For this review, take the finished solid that the model builds, in its own axes (mm). Face numbers are marked on the shaded views. Give positions to 0.01 mm unless a question says otherwise; leave off trailing zeros. Write each loop counter-clockwise with the first axis right and the second up, starting at its lowest first coordinate (ties: lowest second). Pieces come first, ordered by that corner, then holes. Notation, with made-up numbers: M -23,31.25 L -6,31.25 A28 cw -6,58.25 Z; hole C 40.25,52 d5. An arc over 180 degrees is marked long. Write item = value, one per line.
```python
from build123d import *

# Parameters (mm, degrees)
RESSALTO_EXTRUS_O1_DEPTH = 5
ESBO_O2_R                = 2.5
CORTE_EXTRUS_O1_DEPTH    = 218.591641723
RESSALTO_EXTRUS_O2_DEPTH = 30
ESBO_O5_R                = 2.5
CORTE_EXTRUS_O2_DEPTH    = 5
ESBO_O6_R                = 2.5
CORTE_EXTRUS_O3_DEPTH    = 5
CORTE_EXTRUS_O4_DEPTH    = 10


with BuildPart() as part:
    # Esboço1 → Ressalto-extrusão1 (new body)
    with BuildSketch(Plane(origin=(0, 0, 0), x_dir=(1, 0, 0), z_dir=(0, 1, 0))):
        with BuildLine():
            Line((66.608430389, -57.715517241), (91.724137931, -57.715517241))
            ThreePointArc((91.724137931, -57.715517241), (98.795205743, -54.786585053), (101.724137931, -47.715517241))
            Line((101.724137931, -47.715517241), (101.724137931, 182.284482759))
            ThreePointArc((101.724137931, 182.284482759), (98.795205743, 189.35555057), (91.724137931, 192.284482759))
            Line((91.724137931, 192.284482759), (66.608430389, 192.284482759))
            ThreePointArc((66.608430389, 192.284482759), (61.814768465, 191.820595029), (57.199004215, 190.446147187))
            Line((57.199004215, 190.446147187), (-82.685288243, 133.618153375))
            ThreePointArc((-82.685288243, 133.618153375), (-94.015144293, 124.416509464), (-98.275862069, 110.456488947))
            Line((-98.275862069, 110.456488947), (-98.275862069, 24.11247657))
            ThreePointArc((-98.275862069, 24.11247657), (-94.015144293, 10.152456053), (-82.685288243, 0.950812142))
            Line((-82.685288243, 0.950812142), (57.199004215, -55.877181669))
            ThreePointArc((57.199004215, -55.877181669), (61.814768465, -57.251629512), (66.608430389, -57.715517241))
        make_face()
    extrude(amount=RESSALTO_EXTRUS_O1_DEPTH)

    # Esboço2 → Corte-extrusão1 (cut, through all)
    with BuildSketch(Plane(origin=(0, 5, 0), x_dir=(1, 0, 0), z_dir=(0, 1, 0))):
        with Locations(Location((-83.275862069, 102.284482759, 0), (0, 0, 270))):
            Circle(ESBO_O2_R)
        with Locations(Location((86.724137931, 177.284482759, 0), (0, 0, 90))):
            Circle(ESBO_O2_R)
        with Locations(Location((86.724137931, -42.715517241, 0), (0, 0, 270))):
            Circle(ESBO_O2_R)
        with Locations(Location((-83.275862069, 32.284482759, 0), (0, 0, 90))):
            Circle(ESBO_O2_R)
        with BuildLine():
            Line((31.724137931, 107.284482759), (-28.275862069, 107.284482759))
            ThreePointArc((-28.275862069, 107.284482759), (-35.346929881, 104.35555057), (-38.275862069, 97.284482759))
            Line((-38.275862069, 97.284482759), (-38.275862069, 37.284482759))
            ThreePointArc((-38.275862069, 37.284482759), (-35.346929881, 30.213414947), (-28.275862069, 27.284482759))
            Line((-28.275862069, 27.284482759), (31.724137931, 27.284482759))
            ThreePointArc((31.724137931, 27.284482759), (38.795205743, 30.213414947), (41.724137931, 37.284482759))
            Line((41.724137931, 37.284482759), (41.724137931, 97.284482759))
            ThreePointArc((41.724137931, 97.284482759), (38.795205743, 104.35555057), (31.724137931, 107.284482759))
        make_face()
    extrude(amount=-CORTE_EXTRUS_O1_DEPTH, mode=Mode.SUBTRACT)

    # Esboço4 → Ressalto-extrusão2 (add)
    with BuildSketch(Plane(origin=(0, 5, 0), x_dir=(1, 0, 0), z_dir=(0, 1, 0))):
        Polygon((58.224137931, 9.784482759), (-38.275862069, 9.784482759), (-38.275862069, 4.784482759), (63.224137931, 4.784482759), align=None)
        Polygon((58.224137931, 124.784482759), (-38.275862069, 124.784482759), (-38.275862069, 129.784482759), (63.224137931, 129.784482759), align=None)
    extrude(amount=RESSALTO_EXTRUS_O2_DEPTH)

    # Esboço5 → Corte-extrusão2 (cut)
    with BuildSketch(Plane.XY.offset(-4.784482759)):
        with Locations((-30.275862069, 20.836178243)):
            Circle(ESBO_O5_R)
        with Locations((28.724137931, 14.5)):
            Circle(ESBO_O5_R)
    extrude(amount=-CORTE_EXTRUS_O2_DEPTH, mode=Mode.SUBTRACT)

    # Esboço6 → Corte-extrusão3 (cut)
    with BuildSketch(Plane(origin=(0, 0, -129.784482759), x_dir=(-1, 0, 0), z_dir=(0, 0, -1))):
        with Locations((-31.724137931, 14.5)):
            Circle(ESBO_O6_R)
        with Locations((30.275862069, 12.5)):
            Circle(ESBO_O6_R)
    extrude(amount=-CORTE_EXTRUS_O3_DEPTH, mode=Mode.SUBTRACT)

    # Esboço7 → Corte-extrusão4 (cut)
    with BuildSketch(Plane(origin=(0, 5, 0), x_dir=(1, 0, 0), z_dir=(0, 1, 0))):
        with BuildLine():
            Line((76.724137931, 117.284482759), (71.724137931, 117.284482759))
            ThreePointArc((71.724137931, 117.284482759), (64.653070119, 114.35555057), (61.724137931, 107.284482759))
            Line((61.724137931, 107.284482759), (61.724137931, 27.284482759))
            ThreePointArc((61.724137931, 27.284482759), (64.653070119, 20.213414947), (71.724137931, 17.284482759))
            Line((71.724137931, 17.284482759), (76.724137931, 17.284482759))
            ThreePointArc((76.724137931, 17.284482759), (83.795205743, 20.213414947), (86.724137931, 27.284482759))
            Line((86.724137931, 27.284482759), (86.724137931, 107.284482759))
            ThreePointArc((86.724137931, 107.284482759), (83.795205743, 114.35555057), (76.724137931, 117.284482759))
        make_face()
        with BuildLine():
            Line((-58.289420658, 116.784482759), (-63.289420658, 116.784482759))
            ThreePointArc((-63.289420658, 116.784482759), (-70.36048847, 113.85555057), (-73.289420658, 106.784482759))
            Line((-73.289420658, 106.784482759), (-73.289420658, 26.784482759))
            ThreePointArc((-73.289420658, 26.784482759), (-70.36048847, 19.713414947), (-63.289420658, 16.784482759))
            Line((-63.289420658, 16.784482759), (-58.289420658, 16.784482759))
            ThreePointArc((-58.289420658, 16.784482759), (-51.218352846, 19.713414947), (-48.289420658, 26.784482759))
            Line((-48.289420658, 26.784482759), (-48.289420658, 106.784482759))
            ThreePointArc((-48.289420658, 106.784482759), (-51.218352846, 113.85555057), (-58.289420658, 116.784482759))
        make_face()
    extrude(amount=-CORTE_EXTRUS_O4_DEPTH, mode=Mode.SUBTRACT)


solid = part.part
```
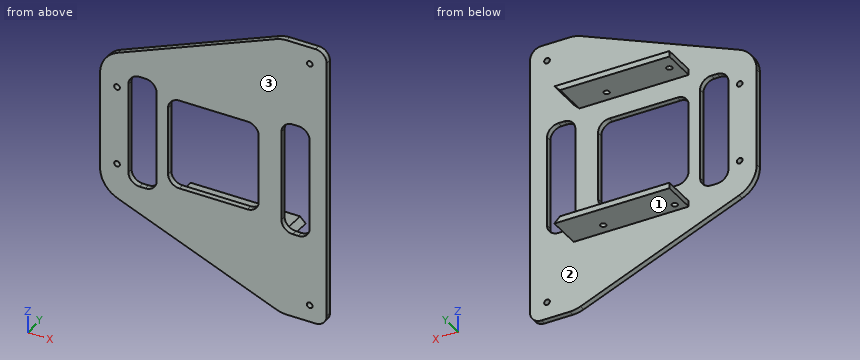
1. We need section B-B, the plane y = 27. Write out the cut boundary in (x, z), then the cut area to 3 significant figures.
Responses:
outline = M -38.28,-129.78 L 63.22,-129.78 L 58.22,-124.78 L -38.28,-124.78 Z; M -38.28,-9.78 L 58.22,-9.78 L 63.22,-4.78 L -38.28,-4.78 Z
area = 990 mm2
2. We need section A-A, the plane z = -84. Write out the cut boundary in (x, y).
Responses:
outline = M -98.28,0 L -73.29,0 L -73.29,5 L -98.28,5 Z; M -48.29,0 L -38.28,0 L -38.28,5 L -48.29,5 Z; M 41.72,0 L 61.72,0 L 61.72,5 L 41.72,5 Z; M 86.72,0 L 101.72,0 L 101.72,5 L 86.72,5 Z
3. We need section D-D, the plane x = -5.5. Write out the cut boundary in (y, z).
Responses:
outline = M 0,-164.97 L 5,-164.97 L 5,-129.78 L 35,-129.78 L 35,-124.78 L 5,-124.78 L 5,-107.28 L 0,-107.28 Z; M 0,-27.28 L 5,-27.28 L 5,-9.78 L 35,-9.78 L 35,-4.78 L 5,-4.78 L 5,30.41 L 0,30.41 Z
4. For line 1 along Z through (x, y) = (-13, 32.5); line 2 along Y through (x, z) = (35, -10); line 3 along Z through (x, y) = (89, 3.5), list the stretches that pass through material, from the lowest coordinate up. Write a range as from..to.
Responses:
line_1 = -129.78..-124.78, -9.78..-4.78
line_2 = 0..5
line_3 = -192.28..-178.32, -176.25..41.68, 43.75..57.72
5. Insertion check: P1, Ø4, axis at x = 86.72, z = -177.28, coming from the +Y side; P2, Ø4, axis at x = 6.5, y = 2, coming from the -Z side; P3, Ø8, axis at x = 20, y = 5.5, coming from the +Z side; P4, Ø4.5, axis at x = 28.72, y = 14.5, coming from the -Z side. Each pin has a flat end and moves straight along its axis. Give the tip position at first contact, or say it passes through.
Responses:
P1 = through
P2 = -170.66
P3 = 42.38
P4 = -129.78
6. We need section C-C, the plane z = -21. Write out the cut boundary in (x, y).
Responses:
outline = M -98.08,0 L -71.45,0 L -71.45,5 L -98.08,5 Z; M -50.13,0 L 63.95,0 L 63.95,5 L -50.13,5 Z; M 84.5,0 L 101.72,0 L 101.72,5 L 84.5,5 Z
7. The part is to be moulded in two halves that separate along Z. For the marked faces 1, 2 and 3, say which applies: +Z half, -Z half, draft (parallel to the pull), parting line (faces both ways), or undercut.
Responses:
face_1 = -Z half
face_2 = undercut
face_3 = draft
